Build history of the part. All positions in model axes, mm. Give positions to 0.01 mm unless a question says otherwise; leave off trailing zeros. Order: outer loops, then holes, each group sorted by start corner. A loop starts at its lowest first (then second) coordinate and runs counter-clockwise, first axis right, second up. Notation, with made-up numbers: (42, -0.5) - (52, -0.5) arc R21 ccw to (52, 11.5) - close; hole circle Ø8 at (8, -24.75). An arc over 180 degrees is marked (long way). Use a Markdown table: item, result. Add a question column.
(1) Flat gauge pin, fed straight in: pin 1 (1 mm diameter, centred on x = 1.5, y = -46, fed in from -Z). Where does the tip first touch, or does it go through?
(2) Wall check: line 1 (Z direction, x = 1.2, y = -12.7) (3 decimals); line 2 (Z direction, x = 0.4, y = -42); line 3 (Z direction, x = 2.2, y = -14.5). Give the ranges that are in metal, low to high.
(3) Slice it at A-A (z = -12.7). Write the cut outline in (x, y) (3 decimals).
(4) Slice it at C-C (z = -63.5). Write the cut outline in (x, y) (3 decimals).
(5) Slice it at B-B (y = -12.7). Write the cut outline in (x, z) (3 decimals).
(6) Slice it at D-D (y = -90.5). Write the cut outline in (x, z) (3 decimals).
Autodesk Inventor part; units mm, degrees
ref_plane "YZ Plane" through (0, 0, 0) normal (1, 0, 0) x (0, 1, 0)
ref_plane "XZ Plane" through (0, 0, 0) normal (0, 1, 0) x (-1, 0, 0)
ref_plane "XY Plane" through (0, 0, 0) normal (0, 0, 1) x (1, 0, 0)
sketch "Sketch1" plane through (0, 0, 0) normal (1, 0, 0) x (0, 1, 0)
  line L0 (0, 0) -> (0, -152.4)
  line L1 (0, -152.4) -> (-25.4, -152.4)
  line L2 (-25.4, -152.4) -> (-101.6, -50.8)
  line L3 (-101.6, -50.8) -> (-101.6, 0)
  circle A0 centre (-63.5, -12.7) radius 3.175
  circle A1 centre (-12.7, -12.7) radius 3.175
  circle A2 centre (-12.7, -76.2) radius 3.175
  circle A3 centre (-12.7, -139.7) radius 3.175
  line L4 (-12.7, 0) -> (-12.7, -152.4) construction
  line L5 (0, -12.7) -> (-101.6, -12.7) construction
  circle A4 centre (-88.9, -38.1) radius 3.175
  circle A5 centre (-38.1, -25.4) radius 4.7625
  line L6 (0, 0) -> (-101.6, 0)
  dimension "d0" = 50.8
  dimension "d1" = 25.4
  dimension "d2" = 101.6
  dimension "d3" = 152.4
  dimension "d4" = 63.5
  dimension "d5" = 63.5
  dimension "d6" = 12.7
  dimension "d8" = 50.8
  dimension "d10" = 12.7
  dimension "d11" = 12.7
  dimension "d13" = 9.525
  dimension "d15" = 6.35
  dimension "d24" = 90
  dimension "d25" = 12.7
  dimension "d26" = 25.4
  dimension "d27" = 152.4
  dimension "d29" = 63.5
extrude "Extrusion1" add sketch "Sketch1" along normal blind 3.175
sketch "Sketch2" plane through (3.175, 0, 0) normal (1, 0, 0) x (0, 0, -1)
  line L0 (50.8, -63.5) -> (50.8, -28.575)
  line L1 (53.975, -25.4) -> (100.5417, -25.4)
  line L2 (102.4467, -31.115) -> (55.88, -66.04)
  line L3 (152.4, 0) -> (0, 0)
  line L4 (0, 0) -> (0, -101.6)
  line L5 (50.8, -101.6) -> (152.4, -25.4)
  arc A0 (50.8, -63.5) -> (55.88, -66.04) centre (53.975, -63.5) ccw
  arc A1 (53.975, -25.4) -> (50.8, -28.575) centre (53.975, -28.575) ccw
  arc A2 (102.4467, -31.115) -> (100.5417, -25.4) centre (100.5417, -28.575) ccw
  line L6 (0, 0) -> (0, -101.6)
  dimension "d18" = 25.4
  dimension "d19" = 25.4
  dimension "d21" = 3.175
  dimension "d28" = 50.8
extrude "Extrusion2" cut sketch "Sketch2" against normal blind 3.175
properties part number "15102898-16-P-0205" material "Aluminum 6061"
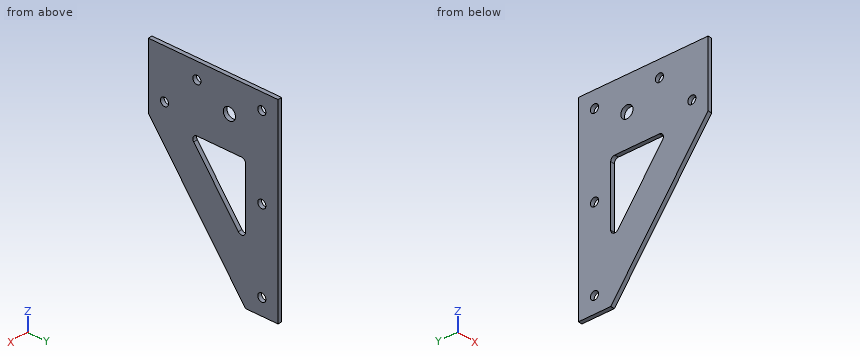
Solution:
| question | item | result |
|---|---|---|
| 1 | pin 1 | z = -125.6 |
| 2 | line 1 | -152.4 to -142.875, -136.525 to -79.375, -73.025 to -15.875, -9.525 to 0 |
| 2 | line 2 | -130.27 to -87.93, -50.8 to -28.13, -22.67 to 0 |
| 2 | line 3 | -152.4 to -142.32, -137.08 to -78.82, -73.58 to -15.32, -10.08 to 0 |
| 3 | outline | (0, -101.6) - (3.175, -101.6) - (3.175, -66.675) - (0, -66.675) - close; (0, -60.325) - (3.175, -60.325) - (3.175, -15.875) - (0, -15.875) - close; (0, -9.525) - (3.175, -9.525) - (3.175, 0) - (0, 0) - close |
| 4 | outline | (0, -92.075) - (3.175, -92.075) - (3.175, -60.325) - (0, -60.325) - close; (0, -25.4) - (3.175, -25.4) - (3.175, 0) - (0, 0) - close |
| 5 | outline | (0, -152.4) - (3.175, -152.4) - (3.175, -142.875) - (0, -142.875) - close; (0, -136.525) - (3.175, -136.525) - (3.175, -79.375) - (0, -79.375) - close; (0, -73.025) - (3.175, -73.025) - (3.175, -15.875) - (0, -15.875) - close; (0, -9.525) - (3.175, -9.525) - (3.175, 0) - (0, 0) - close |
| 6 | outline | (0, -65.6) - (3.175, -65.6) - (3.175, -40.842) - (0, -40.842) - close; (0, -35.358) - (3.175, -35.358) - (3.175, 0) - (0, 0) - close |
